For this review, take the finished solid that the model builds, in its own axes (mm). Coordinates: 2 decimals unless noted, no trailing zeros. Order: outer loops, then holes, each group sorted by start corner. A loop starts at its lowest first (then second) coordinate and runs counter-clockwise, first axis right, second up.
from build123d import *

# Parameters (mm, degrees)
SKETCH090_W     = 445
SKETCH090_H     = 232
PAD027_DEPTH    = 3
SKETCH091_R     = 9.5
POCKET060_DEPTH = 5
FILLET012_R     = 2
POCKET061_DEPTH = 10.001
SKETCH093_R     = 6
SKETCH093_R_2   = 5
POCKET062_DEPTH = 5
SKETCH096_W     = 453.694824
SKETCH096_H     = 509.793549
POCKET065_DEPTH = 5


with BuildPart() as part:
    # Sketch090 → Pad027 (new body)
    with BuildSketch(Plane.XY):
        Rectangle(SKETCH090_W, SKETCH090_H)
    extrude(amount=PAD027_DEPTH)

    # Sketch091 (on Face6 of Pad027) → Pocket060 (cut)
    with BuildSketch(Plane.XY.offset(3)):
        with Locations((-183, 55)):
            Circle(SKETCH091_R)
        with Locations((-183, 33)):
            Circle(SKETCH091_R)
        with Locations((-183, 11)):
            Circle(SKETCH091_R)
        with Locations((-183, -11)):
            Circle(SKETCH091_R)
        with Locations((-183, -33)):
            Circle(SKETCH091_R)
        with Locations((-183, -55)):
            Circle(SKETCH091_R)
        with Locations((-164, 44)):
            Circle(SKETCH091_R)
        with Locations((-164, 22)):
            Circle(SKETCH091_R)
        with Locations((-164, 0)):
            Circle(SKETCH091_R)
        with Locations((-164, -22)):
            Circle(SKETCH091_R)
        with Locations((-164, -44)):
            Circle(SKETCH091_R)
        with Locations((-145, 55)):
            Circle(SKETCH091_R)
        with Locations((-145, 33)):
            Circle(SKETCH091_R)
        with Locations((-145, 11)):
            Circle(SKETCH091_R)
        with Locations((-145, -11)):
            Circle(SKETCH091_R)
        with Locations((-145, -33)):
            Circle(SKETCH091_R)
        with Locations((-145, -55)):
            Circle(SKETCH091_R)
        with Locations((-126, 44)):
            Circle(SKETCH091_R)
        with Locations((-126, 22)):
            Circle(SKETCH091_R)
        with Locations((-126, 0)):
            Circle(SKETCH091_R)
        with Locations((-126, -22)):
            Circle(SKETCH091_R)
        with Locations((-126, -44)):
            Circle(SKETCH091_R)
        with Locations((-107, 55)):
            Circle(SKETCH091_R)
        with Locations((-107, 33)):
            Circle(SKETCH091_R)
        with Locations((-107, 11)):
            Circle(SKETCH091_R)
        with Locations((-107, -11)):
            Circle(SKETCH091_R)
        with Locations((-107, -33)):
            Circle(SKETCH091_R)
        with Locations((-107, -55)):
            Circle(SKETCH091_R)
        with Locations((-88, -44)):
            Circle(SKETCH091_R)
        with Locations((-88, -22)):
            Circle(SKETCH091_R)
        with Locations((-88, 0)):
            Circle(SKETCH091_R)
        with Locations((-88, 22)):
            Circle(SKETCH091_R)
        with Locations((-88, 44)):
            Circle(SKETCH091_R)
        with Locations((-69, 55)):
            Circle(SKETCH091_R)
        with Locations((-69, 33)):
            Circle(SKETCH091_R)
        with Locations((-69, 11)):
            Circle(SKETCH091_R)
        with Locations((-69, -11)):
            Circle(SKETCH091_R)
        with Locations((-69, -33)):
            Circle(SKETCH091_R)
        with Locations((-50, 44)):
            Circle(SKETCH091_R)
        with Locations((-50, 22)):
            Circle(SKETCH091_R)
        with Locations((-50, 0)):
            Circle(SKETCH091_R)
        with Locations((-50, -22)):
            Circle(SKETCH091_R)
        with Locations((-50, -44)):
            Circle(SKETCH091_R)
        with Locations((-69, -55)):
            Circle(SKETCH091_R)
        with Locations((-31, 55)):
            Circle(SKETCH091_R)
        with Locations((-31, 33)):
            Circle(SKETCH091_R)
        with Locations((-31, 11)):
            Circle(SKETCH091_R)
        with Locations((-31, -11)):
            Circle(SKETCH091_R)
        with Locations((-31, -33)):
            Circle(SKETCH091_R)
        with Locations((-31, -55)):
            Circle(SKETCH091_R)
        with Locations((-12, -44)):
            Circle(SKETCH091_R)
        with Locations((-12, -22)):
            Circle(SKETCH091_R)
        with Locations((-12, 0)):
            Circle(SKETCH091_R)
        with Locations((-12, 22)):
            Circle(SKETCH091_R)
        with Locations((-12, 44)):
            Circle(SKETCH091_R)
        with Locations((7, 55)):
            Circle(SKETCH091_R)
        with Locations((7, 33)):
            Circle(SKETCH091_R)
        with Locations((7, 11)):
            Circle(SKETCH091_R)
        with Locations((7, -11)):
            Circle(SKETCH091_R)
        with Locations((7, -33)):
            Circle(SKETCH091_R)
        with Locations((7, -55)):
            Circle(SKETCH091_R)
        with Locations((26, -44)):
            Circle(SKETCH091_R)
        with Locations((26, -22)):
            Circle(SKETCH091_R)
        with Locations((26, 0)):
            Circle(SKETCH091_R)
        with Locations((26, 22)):
            Circle(SKETCH091_R)
        with Locations((26, 44)):
            Circle(SKETCH091_R)
        with Locations((45, 55)):
            Circle(SKETCH091_R)
        with Locations((45, 33)):
            Circle(SKETCH091_R)
        with Locations((45, 11)):
            Circle(SKETCH091_R)
        with Locations((45, -11)):
            Circle(SKETCH091_R)
        with Locations((64, 0)):
            Circle(SKETCH091_R)
        with Locations((64, 22)):
            Circle(SKETCH091_R)
        with Locations((64, 44)):
            Circle(SKETCH091_R)
        with Locations((45, -33)):
            Circle(SKETCH091_R)
        with Locations((45, -55)):
            Circle(SKETCH091_R)
        with Locations((64, -44)):
            Circle(SKETCH091_R)
        with Locations((64, -22)):
            Circle(SKETCH091_R)
        with Locations((83, 55)):
            Circle(SKETCH091_R)
        with Locations((83, 33)):
            Circle(SKETCH091_R)
        with Locations((83, 11)):
            Circle(SKETCH091_R)
        with Locations((83, -11)):
            Circle(SKETCH091_R)
        with Locations((83, -33)):
            Circle(SKETCH091_R)
        with Locations((83, -55)):
            Circle(SKETCH091_R)
        with Locations((102, 44)):
            Circle(SKETCH091_R)
        with Locations((102, 22)):
            Circle(SKETCH091_R)
        with Locations((102, 0)):
            Circle(SKETCH091_R)
        with Locations((102, -22)):
            Circle(SKETCH091_R)
        with Locations((102, -44)):
            Circle(SKETCH091_R)
        with Locations((121, 55)):
            Circle(SKETCH091_R)
        with Locations((121, 33)):
            Circle(SKETCH091_R)
        with Locations((121, 11)):
            Circle(SKETCH091_R)
        with Locations((121, -11)):
            Circle(SKETCH091_R)
        with Locations((121, -33)):
            Circle(SKETCH091_R)
        with Locations((121, -55)):
            Circle(SKETCH091_R)
        with Locations((140, 44)):
            Circle(SKETCH091_R)
        with Locations((140, 22)):
            Circle(SKETCH091_R)
        with Locations((140, 0)):
            Circle(SKETCH091_R)
        with Locations((140, -22)):
            Circle(SKETCH091_R)
        with Locations((140, -44)):
            Circle(SKETCH091_R)
        with Locations((159, 55)):
            Circle(SKETCH091_R)
        with Locations((159, 33)):
            Circle(SKETCH091_R)
        with Locations((159, 11)):
            Circle(SKETCH091_R)
        with Locations((159, -11)):
            Circle(SKETCH091_R)
        with Locations((159, -33)):
            Circle(SKETCH091_R)
        with Locations((159, -55)):
            Circle(SKETCH091_R)
        with Locations((-164, 66)):
            Circle(SKETCH091_R)
        with Locations((-126, 66)):
            Circle(SKETCH091_R)
        with Locations((-88, 66)):
            Circle(SKETCH091_R)
        with Locations((-50, 66)):
            Circle(SKETCH091_R)
        with Locations((-12, 66)):
            Circle(SKETCH091_R)
        with Locations((26, 66)):
            Circle(SKETCH091_R)
        with Locations((64, 66)):
            Circle(SKETCH091_R)
        with Locations((102, 66)):
            Circle(SKETCH091_R)
        with Locations((140, 66)):
            Circle(SKETCH091_R)
        with Locations((-164, -66)):
            Circle(SKETCH091_R)
        with Locations((-126, -66)):
            Circle(SKETCH091_R)
        with Locations((-88, -66)):
            Circle(SKETCH091_R)
        with Locations((-50, -66)):
            Circle(SKETCH091_R)
        with Locations((-12, -66)):
            Circle(SKETCH091_R)
        with Locations((26, -66)):
            Circle(SKETCH091_R)
        with Locations((64, -66)):
            Circle(SKETCH091_R)
        with Locations((102, -66)):
            Circle(SKETCH091_R)
        with Locations((140, -66)):
            Circle(SKETCH091_R)
        with Locations((178, 66)):
            Circle(SKETCH091_R)
        with Locations((178, 44)):
            Circle(SKETCH091_R)
        with Locations((178, 22)):
            Circle(SKETCH091_R)
        with Locations((178, 0)):
            Circle(SKETCH091_R)
        with Locations((178, -22)):
            Circle(SKETCH091_R)
        with Locations((178, -44)):
            Circle(SKETCH091_R)
        with Locations((178, -66)):
            Circle(SKETCH091_R)
    extrude(amount=-POCKET060_DEPTH, mode=Mode.SUBTRACT)

    # Fillet012
    fillet012_edges = [part.edges().sort_by_distance(p)[0] for p in [
        (-222.5, -116, 1.5),
        (222.5, -116, 1.5),
        (222.5, 116, 1.5),
        (-222.5, 116, 1.5),
    ]]
    fillet(fillet012_edges, radius=FILLET012_R)

    # Sketch092 → Pocket061 (cut, through all)
    with BuildSketch(Plane.XY.offset(10)):
        Polygon((188.873749, -62), (214.664444, -62), (214.664444, 62), (188.873749, 62), (188.873749, 11.724954), (183.462372, 4.250606), (183.462372, -4.752587), (188.873749, -11.972128), align=None)
    extrude(amount=-POCKET061_DEPTH, mode=Mode.SUBTRACT)

    # Sketch093 (on Face2 of Pocket061) → Pocket062 (cut)
    with BuildSketch(Plane(origin=(0, 0, 0), x_dir=(1, 0, 0), z_dir=(0, 0, -1))):
        with Locations((213.5, 50)):
            Circle(SKETCH093_R)
        with Locations((213.5, -50)):
            Circle(SKETCH093_R)
        with Locations((-213.5, 50)):
            Circle(SKETCH093_R)
        with Locations((-213.5, -50)):
            Circle(SKETCH093_R)
        with Locations((-163.5, 90)):
            Circle(SKETCH093_R_2)
        with Locations((-25.5, 90)):
            Circle(SKETCH093_R_2)
        with Locations((163.5, 90)):
            Circle(SKETCH093_R_2)
        with Locations((163.5, -90)):
            Circle(SKETCH093_R_2)
        with Locations((-25.5, -90)):
            Circle(SKETCH093_R_2)
        with Locations((-163.5, -90)):
            Circle(SKETCH093_R_2)
    extrude(amount=-POCKET062_DEPTH, mode=Mode.SUBTRACT)

    # Sketch096 (on Face5 of Pocket062) → Pocket065 (cut)
    with BuildSketch(Plane.XY.offset(3)):
        with Locations((196.847412, -60.920081)):
            Rectangle(SKETCH096_W, SKETCH096_H)
    extrude(amount=-POCKET065_DEPTH, mode=Mode.SUBTRACT)


with BuildPart() as part_1:
    # Body023 placement: moved
    add(part.part.moved(Location((0, 0, -3))))


solid = part_1.part
1. Take a section at C-C, the plane x = -50. Give the number of separate pieces and of enclosed holes in the cut face, plus the area to 3 significant figures.
Answer below:
separate pieces: 8
enclosed holes: 0
area: 297 mm2
2. Clearance check with a flat-ended pin moving along its axis: pin 1 Ø11.5 at (x, y) = (-163.5, -90) entering from -Z. State where the tip first meets the part, or that it passes through.
Answer below:
pin 1: stops at z = -3
3. The part is to be moulded in two halves that separate along Y. For faces 1 (the face through (-158.89, 74.01, -1.48)), 2 (the face through (-149, 2, -3)), 3 (the face through (-95, -37.58, -1.48)), say which applies: +Y half, -Y half, draft (parallel to the pull), parting line (faces both ways), or undercut.
Answer below:
face 1: undercut
face 2: draft
face 3: undercut
4. Take a section at A-A, the plane x = -107. Give the boundary of the cut face in (y, z).
Answer below:
outline: (-116, -3) - (-64.5, -3) - (-64.5, 0) - (-116, 0) - close; (-45.5, -3) - (-42.5, -3) - (-42.5, 0) - (-45.5, 0) - close; (-23.5, -3) - (-20.5, -3) - (-20.5, 0) - (-23.5, 0) - close; (-1.5, -3) - (1.5, -3) - (1.5, 0) - (-1.5, 0) - close; (20.5, -3) - (23.5, -3) - (23.5, 0) - (20.5, 0) - close; (42.5, -3) - (45.5, -3) - (45.5, 0) - (42.5, 0) - close; (64.5, -3) - (116, -3) - (116, 0) - (64.5, 0) - close
5. To check wall thickness, follow L1, parallel to X at y = 1, z = -2.05; L2, parallel to X at y = -68, z = -0.6. State the ranges of each line that lie inside material, in increasing order.
Answer below:
L1: x = -222.5 to -173.45, -154.55 to -135.45, -116.55 to -97.45, -78.55 to -59.45, -40.55 to -30
L2: x = -222.5 to -173.29, -154.71 to -135.29, -116.71 to -97.29, -78.71 to -59.29, -40.71 to -30
6. Take a section at B-B, the plane y = 70. Give the boundary of the cut face in (x, z).
Answer below:
outline: (-222.5, -3) - (-172.62, -3) - (-172.62, 0) - (-222.5, 0) - close; (-155.38, -3) - (-134.62, -3) - (-134.62, 0) - (-155.38, 0) - close; (-117.38, -3) - (-96.62, -3) - (-96.62, 0) - (-117.38, 0) - close; (-79.38, -3) - (-58.62, -3) - (-58.62, 0) - (-79.38, 0) - close; (-41.38, -3) - (-30, -3) - (-30, 0) - (-41.38, 0) - close
